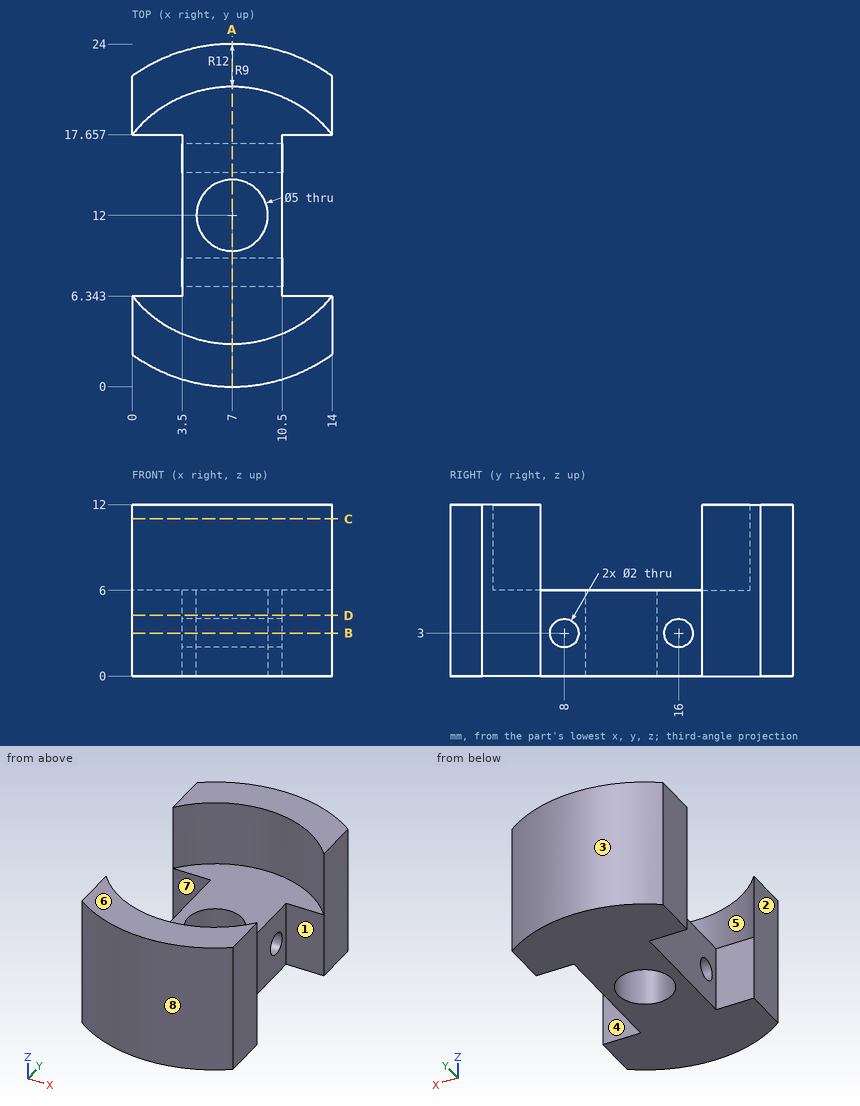
Input: dimensioned drawing with shaded views. Units: mm. Origin: part minimum x, y, z. A direction names the side the tool comes from. Coordinates: 2 decimals unless noted, no trailing zeros. Loops run counter-clockwise (first coordinate to the right, second up) from the corner with the lowest first, then second, coordinate; pieces in that order, holes last. Notation, with made-up numbers: M 43.5,-19.5 L 95.5,-19.5 A17 cw 95.5,0.5 Z; hole C -34,-13 d4. An arc over 180 degrees is marked long. Use a Markdown table: item, result. Add a question column.
Q1. Section query B-B, the plane z = 3. Return loops of the section in (x, y).
Q2. Draft query along Y for the marked faces 1, 2 and 3. Return one class per face: pulls with the +Y half, pulls with the -Y half, needs draft (parallel to the pull), parting line crosses it, or undercut.
Q3. Section query D-D, the plane z = 4.25. Return loops of the section in (x, y), and give its area (3 significant figures).
Q4. Access query for the marked faces 4, 5, 6, 7 and 8. Directions: +Z, -Z, +X, -X, +Y, -Y. A direction counts if a zero-diameter tool reaches every point of the face in a straight line with its end or side. Return the directions, or none.
Q5. Section query A-A, the plane x = 7. Return loops of the section in (y, z).
Q6. Material intervals for L1, parallel to Y at x = 7.25, z = 11.25; L2, parallel to Y at x = 8, z = 3; L3, parallel to Y at x = 1, z = 9, sorted ascending.
Q7. First-contact query: pin 1 (3 mm diameter, centred on x = 12, z = 4, fed in from +Y); pin 2 (2 mm diameter, centred on y = 16.5, z = 4.5, fed in from -X); pin 3 (1.8 mm diameter, centred on x = 1.5, z = 4, fed in from +Y). Flat tips, straight axial feed; report the tip coordinate or a pass-through.
Q8. Section query C-C, the plane z = 11. Return loops of the section in (x, y).
Result:
| question | item | result |
|---|---|---|
| 1 | outline | M 0,2.25 A12 ccw 14,2.25 L 14,6.34 L 10.5,6.34 L 10.5,7 L 3.5,7 L 3.5,6.34 L 0,6.34 Z; M 0,17.66 L 3.5,17.66 L 3.5,17 L 10.5,17 L 10.5,17.66 L 14,17.66 L 14,21.75 A12 ccw 0,21.75 Z; M 3.5,9 L 10.5,9 L 10.5,15 L 3.5,15 Z; hole C 7,12 d5 |
| 2 | face 1 | undercut |
| 2 | face 2 | needs draft |
| 2 | face 3 | pulls with the +Y half |
| 3 | outline | M 0,2.25 A12 ccw 14,2.25 L 14,6.34 L 10.5,6.34 L 10.5,17.66 L 14,17.66 L 14,21.75 A12 ccw 0,21.75 L 0,17.66 L 3.5,17.66 L 3.5,6.34 L 0,6.34 Z; hole C 7,12 d5 |
| 3 | area | 217 mm2 |
| 4 | face 4 | +Z, -Z, +X |
| 4 | face 5 | +Z |
| 4 | face 6 | +Z, +X, -X, +Y, -Y |
| 4 | face 7 | +Z, -Z, -X |
| 4 | face 8 | +Z, -Z, -Y |
| 5 | outline | M 0,0 L 9.5,0 L 9.5,6 L 3,6 L 3,12 L 0,12 Z; M 14.5,0 L 24,0 L 24,12 L 21,12 L 21,6 L 14.5,6 Z; hole C 8,3 d2; hole C 16,3 d2 |
| 6 | L1 | y = 0 to 3, 21 to 24 |
| 6 | L2 | y = 0.04 to 7, 9 to 9.71, 14.29 to 15, 17 to 23.96 |
| 6 | L3 | y = 1.61 to 5.29, 18.71 to 22.39 |
| 7 | pin 1 | stops at y = 23.48 |
| 7 | pin 2 | stops at x = 3.5 |
| 7 | pin 3 | stops at y = 23.08 |
| 8 | outline | M 0,2.25 A12 ccw 14,2.25 L 14,6.34 A9 cw 0,6.34 Z; M 0,17.66 A9 cw 14,17.66 L 14,21.75 A12 ccw 0,21.75 Z |
